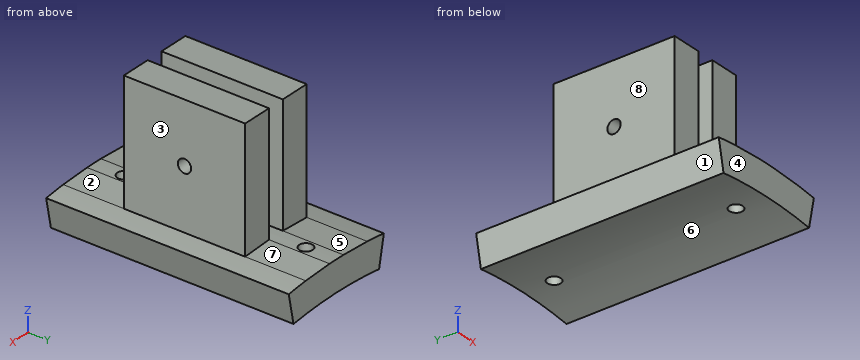
from build123d import *

# Parameters (mm, degrees)
BOSS_EXTRUDE1_DEPTH      = 25.4
SKETCH3_R                = 1.397
CUT_EXTRUDE2_DEPTH       = 25.4
BOSS_EXTRUDE2_DEPTH      = 12.7
BOSS_EXTRUDE2_DEPTH_BACK = 38.1
CUT_EXTRUDE3_REACH       = 34.125
SKETCH5_R                = 1.397


with BuildPart() as part:
    # Sketch1 → Boss-Extrude1 (new body)
    with BuildSketch(Plane(origin=(0, 0, 0), x_dir=(1, 0, 0), z_dir=(0, 1, 0))):
        with BuildLine():
            Line((-8.255, -94.891609086), (-8.255, -120.291609086))
            Line((-8.255, -120.291609086), (-1.905, -120.291609086))
            Line((-1.905, -120.291609086), (-1.905, -95.230948095))
            ThreePointArc((-1.905, -95.230948095), (-0.063511871, -95.249978825), (1.778, -95.233403888))
            Line((1.778, -95.233403888), (1.778, -120.291609086))
            Line((1.778, -120.291609086), (8.128, -120.291609086))
            Line((8.128, -120.291609086), (8.128, -94.902571704))
            ThreePointArc((8.128, -94.902571704), (10.398183486, -94.680728135), (12.662403805, -94.404586911))
            Line((12.662403805, -94.404586911), (11.398535202, -88.166225933))
            ThreePointArc((11.398535202, -88.166225933), (0, -88.9), (-11.398535202, -88.166225933))
            Line((-11.398535202, -88.166225933), (-12.662403805, -94.404586911))
            ThreePointArc((-12.662403805, -94.404586911), (-10.461536366, -94.673749038), (-8.255, -94.891609086))
        make_face()
    extrude(amount=BOSS_EXTRUDE1_DEPTH)

    # Sketch3 → Cut-Extrude2 (cut)
    with BuildSketch(Plane.ZY.offset(8.255)):
        with Locations((107.591609086, 12.7)):
            Circle(SKETCH3_R)
    extrude(amount=-CUT_EXTRUDE2_DEPTH, mode=Mode.SUBTRACT)

    # Sketch4 → Boss-Extrude2 (add, two sides)
    with BuildSketch(Plane(origin=(0, 25.4, 0), x_dir=(1, 0, 0), z_dir=(0, 1, 0))) as boss_extrude2_sk:
        with BuildLine():
            Line((1.778, -95.233403888), (8.128, -94.902571704))
            ThreePointArc((8.128, -94.902571704), (10.398183486, -94.680728135), (12.662403805, -94.404586911))
            Line((12.662403805, -94.404586911), (11.398535202, -88.166225933))
            ThreePointArc((11.398535202, -88.166225933), (0, -88.9), (-11.398535202, -88.166225933))
            Line((-11.398535202, -88.166225933), (-12.662403805, -94.404586911))
            ThreePointArc((-12.662403805, -94.404586911), (-10.461536366, -94.673749038), (-8.255, -94.891609086))
            Line((-8.255, -94.891609086), (-1.905, -95.230948095))
            ThreePointArc((-1.905, -95.230948095), (-0.063511871, -95.249978825), (1.778, -95.233403888))
        make_face()
    extrude(amount=BOSS_EXTRUDE2_DEPTH)
    extrude(boss_extrude2_sk.sketch, amount=-BOSS_EXTRUDE2_DEPTH_BACK)

    # Sketch5 → Cut-Extrude3 (cut, up to next)
    with BuildSketch(Plane.XY.offset(120.291609086), mode=Mode.PRIVATE) as cut_extrude3_sk1:
        with Locations((0, 31.75)):
            Circle(SKETCH5_R)
    cut_extrude3_tool1 = extrude(cut_extrude3_sk1.sketch, amount=-CUT_EXTRUDE3_REACH, mode=Mode.PRIVATE) & part.part
    add(cut_extrude3_tool1.solids().sort_by_distance((0, 31.75, 120.291609))[0], mode=Mode.SUBTRACT)
    # Sketch5 → Cut-Extrude3 (cut, up to next)
    with BuildSketch(Plane.XY.offset(120.291609086), mode=Mode.PRIVATE) as cut_extrude3_sk2:
        with Locations((0, -6.35)):
            Circle(SKETCH5_R)
    cut_extrude3_tool2 = extrude(cut_extrude3_sk2.sketch, amount=-CUT_EXTRUDE3_REACH, mode=Mode.PRIVATE) & part.part
    add(cut_extrude3_tool2.solids().sort_by_distance((0, -6.35, 120.291609))[0], mode=Mode.SUBTRACT)


solid = part.part
The listing builds one solid part. Answer for the finished solid, in the listing's coordinates (mm). Face numbers are marked on the shaded views. A direction names the side the tool comes from. Give positions to 0.01 mm unless a question says otherwise; leave off trailing zeros. Write each loop counter-clockwise with the first axis right and the second up, starting at its lowest first coordinate (ties: lowest second). Pieces come first, ordered by that corner, then holes. Notation, with made-up numbers: (43.5, 70) -> (83.5, 70) arc R27 cw to (83.5, 105) -> close; hole circle Ø1 at (-24.75, 51). An arc over 180 degrees is marked (long way). Use a Markdown table: item, result.
(1) Find the intervals of material crossed by probe 1 along Y at (x, z) = (0, 90.5); probe 2 along X at (y, z) = (16.5, 112) (3 decimals); probe 3 along Z at (x, y) = (-0.75, 11), in increasing order. Write a range as from..to.
Return value:
| item | result |
|---|---|
| probe 1 | -12.7..-7.75, -4.95..30.35, 33.15..38.1 |
| probe 2 | -8.255..-1.905, 1.778..8.128 |
| probe 3 | 88.9..95.25 |
(2) Section B-B, the plane z = 100 is taken. Determine the outline of the cut face in (x, y) (3 decimals), then the cut area to 3 significant figures.
Return value:
| item | result |
|---|---|
| outline | (-8.255, 0) -> (-1.905, 0) -> (-1.905, 25.4) -> (-8.255, 25.4) -> close; (1.778, 0) -> (8.128, 0) -> (8.128, 25.4) -> (1.778, 25.4) -> close |
| area | 323 mm2 |
(3) Flat-ended cylindrical pins translate along their axes: P1, Ø1.9, axis at x = -5, z = 110.5, coming from the +Y side; P2, Ø12, axis at y = 26, z = 109, coming from the -X side (3 decimals); P3, Ø6, axis at x = 3.5, z = 112.5, coming from the -Y side. Find the tip coordinate at first contact, or state that the pin passes through.
Return value:
| item | result |
|---|---|
| P1 | y = 25.4 |
| P2 | x = -8.255 |
| P3 | y = 0 |
(4) Determine the mould class of the marked faces 6, 7 and 8 for opening direction X: released by +X, released by -X, zero draft, split by the parting line, or undercut.
Return value:
| item | result |
|---|---|
| face 6 | undercut |
| face 7 | released by +X |
| face 8 | released by -X |
(5) Section C-C, the plane x = 0 is taken. Determine the outline of the cut face in (y, z).
Return value:
| item | result |
|---|---|
| outline | (-12.7, 88.9) -> (-7.75, 88.9) -> (-7.75, 95.25) -> (-12.7, 95.25) -> close; (-4.95, 88.9) -> (30.35, 88.9) -> (30.35, 95.25) -> (-4.95, 95.25) -> close; (33.15, 88.9) -> (38.1, 88.9) -> (38.1, 95.25) -> (33.15, 95.25) -> close |
(6) Section A-A, the plane y = 12.7 is taken. Determine the outline of the cut face in (x, z) (3 decimals), then the cut area to 3 significant figures.
Return value:
| item | result |
|---|---|
| outline | (-12.662, 94.405) -> (-11.399, 88.166) arc R88.9 cw to (11.399, 88.166) -> (12.662, 94.405) arc R95.25 ccw to (8.128, 94.903) -> (8.128, 106.195) -> (1.778, 106.195) -> (1.778, 95.233) arc R95.25 ccw to (-1.905, 95.231) -> (-1.905, 106.195) -> (-8.255, 106.195) -> (-8.255, 94.892) arc R95.25 ccw to start; (-8.255, 108.989) -> (-1.905, 108.989) -> (-1.905, 120.292) -> (-8.255, 120.292) -> close; (1.778, 108.989) -> (8.128, 108.989) -> (8.128, 120.292) -> (1.778, 120.292) -> close |
| area | 438 mm2 |
(7) Section D-D, the plane y = 34 is taken. Determine the outline of the cut face in (x, z) (3 decimals), then the cut area to 3 significant figures.
Return value:
| item | result |
|---|---|
| outline | (-12.662, 94.405) -> (-11.399, 88.166) arc R88.9 cw to (11.399, 88.166) -> (12.662, 94.405) arc R95.25 ccw to (8.128, 94.903) -> (1.778, 95.233) arc R95.25 ccw to (-1.905, 95.231) -> (-8.255, 94.892) arc R95.25 ccw to start |
| area | 153 mm2 |
(8) For the marked faces 1, 2, 3, 4 and 5, determine the directions among +Z, -Z, +X, -X, +Y, -Y from which every point of the face is accessible in a straight line to the end or side of a thin tool.
Return value:
| item | result |
|---|---|
| face 1 | -Z, -X, +Y, -Y |
| face 2 | +Z, +X, -Y |
| face 3 | +Z, +X, +Y, -Y |
| face 4 | +Z, -Z, +X, -X, -Y |
| face 5 | +Z, -X, +Y |
